The listing builds one solid part. Answer for the finished solid, in the listing's coordinates (mm). Face numbers are marked on the shaded views. A direction names the side the tool comes from. Round coordinates to 2 decimals unless told otherwise and drop trailing zeros. Order: outer loops, then holes, each group sorted by start corner. A loop starts at its lowest first (then second) coordinate and runs counter-clockwise, first axis right, second up. Notation, with made-up numbers: (78, 81) - (87, 81) arc R10 ccw to (87, 99) - close; hole circle Ø6 at (-39, -33). An arc over 180 degrees is marked (long way). Write item = value, one per line.
from build123d import *

# Parameters (mm, degrees)
BOSS_EXTRUDE1_DEPTH = 82
CUT_EXTRUDE1_DEPTH  = 105
SKETCH3_W           = 23
SKETCH3_H           = 43
CUT_EXTRUDE2_DEPTH  = 28
CUT_EXTRUDE3_DEPTH  = 32
CUT_EXTRUDE4_DEPTH  = 32
SKETCH7_W           = 12.805148614
SKETCH7_H           = 2.400001526
CUT_EXTRUDE5_DEPTH  = 89
SKETCH8_W           = 27.756866021
SKETCH8_H           = 1.710281704
CUT_EXTRUDE6_DEPTH  = 89


with BuildPart() as part:
    # Sketch1 → Boss-Extrude1 (new body)
    with BuildSketch(Plane(origin=(0, 0, 0), x_dir=(1, 0, 0), z_dir=(0, 1, 0))):
        with BuildLine():
            Line((-21.9286378, 20.529965557), (30.819410356, 20.529965557))
            Line((30.819410356, 20.529965557), (30.819410356, 8.269460429))
            ThreePointArc((30.819410356, 8.269460429), (29.737157279, 6.984989328), (28.898083391, 5.52996605))
            Line((28.898083391, 5.52996605), (24.81959218, 5.52996605))
            Line((24.81959218, 5.52996605), (14.820019426, -17.47003395))
            Line((14.820019426, -17.47003395), (3.320446672, -17.47003395))
            ThreePointArc((3.320446672, -17.47003395), (-2.977277813, -22.983126936), (-11.218310652, -24.446310348))
            ThreePointArc((-11.218310652, -24.446310348), (-19.829053504, -21.990642561), (-25.924914656, -15.432009048))
            Line((-25.924914656, -15.432009048), (-26.328479109, -14.47003395))
            Line((-26.328479109, -14.47003395), (-25.288623152, -0.544399566))
            Line((-25.288623152, -0.544399566), (-24.844287214, 3.45451706))
            Line((-24.844287214, 3.45451706), (-24.102893172, 7.451406174))
            Line((-24.102893172, 7.451406174), (-23.328601179, 10.529965096))
            Line((-23.328601179, 10.529965096), (-22.928576765, 16.529967242))
            Line((-22.928576765, 16.529967242), (-22.928576765, 18.529964858))
            Line((-22.928576765, 18.529964858), (-21.9286378, 20.529965557))
        make_face()
    extrude(amount=BOSS_EXTRUDE1_DEPTH)

    # Sketch2 → Cut-Extrude1 (cut)
    with BuildSketch(Plane.XZ):
        Polygon((-18.173439963, -16.784486826), (-18.173439963, 15.715513413), (-3.173989279, 15.715513413), (-3.173989279, 13.315508549), (9.57552244, 13.315508549), (9.57552244, -14.3844853), (-3.173989279, -14.3844853), (-3.173989279, -16.784486826), align=None)
    extrude(amount=-CUT_EXTRUDE1_DEPTH, mode=Mode.SUBTRACT)

    # Sketch3 → Cut-Extrude2 (cut)
    with BuildSketch(Plane(origin=(40, 0, 0), x_dir=(0, 0, -1), z_dir=(1, 0, 0))):
        with Locations((-5.976477548, 53.208460465)):
            Rectangle(SKETCH3_W, SKETCH3_H)
    extrude(amount=-CUT_EXTRUDE2_DEPTH, mode=Mode.SUBTRACT)

    # Sketch5 → Cut-Extrude3 (cut)
    with BuildSketch(Plane.XZ):
        Polygon((14.820019426, 17.47003395), (24.81959218, -5.52996605), (14.820019426, -5.52996605), align=None)
    extrude(amount=-CUT_EXTRUDE3_DEPTH, mode=Mode.SUBTRACT)

    # Sketch6 → Cut-Extrude4 (cut)
    with BuildSketch(Plane.XZ):
        Polygon((27.668053931, -5.521484947), (27.668053931, -9.376004197), (27.668053931, -18.376004197), (9.668053931, -18.376004197), (9.57552244, -14.3844853), (9.57552244, 13.315508549), (3.20076658, 13.315508549), (3.320446672, 17.47003395), (14.820019426, 17.47003395), (14.820019426, -5.52996605), align=None)
    extrude(amount=-CUT_EXTRUDE4_DEPTH, mode=Mode.SUBTRACT)

    # Sketch7 → Cut-Extrude5 (cut)
    with BuildSketch(Plane.XZ):
        with Locations((3.228585028, -15.584486063)):
            Rectangle(SKETCH7_W, SKETCH7_H)
    extrude(amount=-CUT_EXTRUDE5_DEPTH, mode=Mode.SUBTRACT)

    # Sketch8 → Cut-Extrude6 (cut)
    with BuildSketch(Plane.XZ):
        with Locations((-4.247273675, -17.639627678)):
            Rectangle(SKETCH8_W, SKETCH8_H)
    extrude(amount=-CUT_EXTRUDE6_DEPTH, mode=Mode.SUBTRACT)


solid = part.part
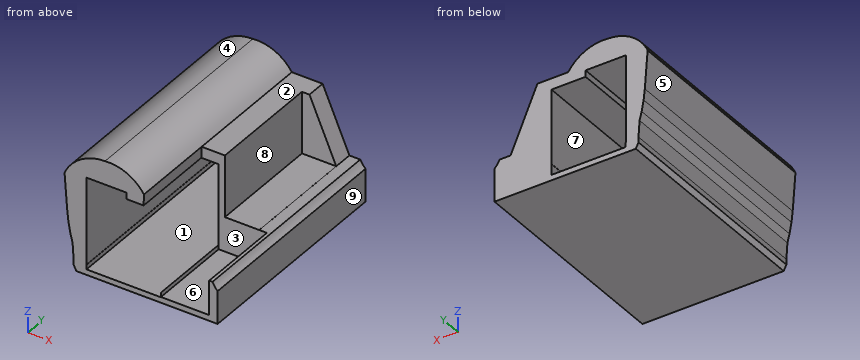
Q1. Find the intervals of material crossed by line 1 (Z direction, x = 24, y = 20.5); line 2 (X direction, y = 37, z = -10); line 3 (X direction, y = 36, z = -12.5), in increasing order. Write a range as from..to.
Model answer:
line_1 = -20.53..-18.38
line_2 = -23.46..-18.17, 9.58..30.82
line_3 = -23.2..-18.17, 9.58..30.82
Q2. For the marked faces 5, 6, 7, 8 and 9, determine the directions among +Z, -Z, +X, -X, +Y, -Y from which every point of the face is accessible in a straight line to the end or side of a thin tool.
Model answer:
face_5 = -Z, -X, +Y, -Y
face_6 = +Z, -Y
face_7 = +Y, -Y
face_8 = +Z, +X, -Y
face_9 = +Z, -Z, +X, +Y, -Y
Q3. Determine the mould class of the marked faces 1, 2, 3 and 4 for opening direction X: released by +X, released by -X, zero draft, split by the parting line, or undercut.
Model answer:
face_1 = undercut
face_2 = zero draft
face_3 = undercut
face_4 = released by -X
Q4. Section B-B on z = 8.5 is taken. Determine the outline of the cut face in (x, y), then the cut area to 3 significant figures.
Model answer:
outline = (-25.88, 0) - (-18.17, 0) - (-18.17, 82) - (-25.88, 82) - close; (9.58, 32) - (12, 32) - (12, 74.71) - (18.72, 74.71) - (18.72, 82) - (9.58, 82) - close
area = 802 mm^2
Q5. Flat-ended cylindrical pins translate along their axes: P1, Ø12, axis at x = 9.5, z = -4.5, coming from the -Y side; P2, Ø8, axis at x = 0, y = 33.5, coming from the +Z side; P3, Ø11.5, axis at y = 54, z = 2.5, coming from the +X side. Find the tip coordinate at first contact, or state that the pin passes through.
Model answer:
P1 = 32
P2 = 23.43
P3 = 12
Q6. Section D-D on y = 19.5 is taken. Determine the outline of the cut face in (x, z), then the cut area to 3 significant figures.
Model answer:
outline = (-26.33, 14.47) - (-25.29, 0.54) - (-24.84, -3.45) - (-24.1, -7.45) - (-23.33, -10.53) - (-22.93, -16.53) - (-22.93, -18.53) - (-21.93, -20.53) - (30.82, -20.53) - (30.82, -8.27) arc R9.5 cw to (28.9, -5.53) - (27.67, -5.53) - (27.67, -18.38) - (9.67, -18.38) - (9.63, -16.78) - (9.63, -18.49) - (-18.13, -18.49) - (-18.13, -16.78) - (-18.17, -16.78) - (-18.17, 15.72) - (-3.17, 15.72) - (-3.17, 13.32) - (3.2, 13.32) - (3.32, 17.47) arc R15.6 ccw to (-11.22, 24.45) arc R16.66 ccw to (-25.92, 15.43) - close
area = 580 mm^2
Q7. Section C-C on x = -14 is taken. Determine the outline of the cut face in (y, z), then the cut area to 3 significant figures.
Model answer:
outline = (0, -20.53) - (82, -20.53) - (82, -18.49) - (0, -18.49) - close; (0, 15.72) - (82, 15.72) - (82, 24.2) - (0, 24.2) - close
area = 862 mm^2
